Design review of the part built by this model. Coordinates are the model's own, in mm. A direction names the side the tool comes from. Give positions to 0.01 mm unless a question says otherwise; leave off trailing zeros. Loops run counter-clockwise (first coordinate to the right, second up) from the corner with the lowest first, then second, coordinate; pieces in that order, holes last. Notation, with made-up numbers: (23, 20.5) - (80, 20.5) arc R35 ccw to (80, 52.5) - close; hole circle Ø5 at (60.5, -40). An arc over 180 degrees is marked (long way). Write each question's results on one line, items separated by ' | '.
```python
from build123d import *

# Parameters (mm, degrees)
SKETCH1_R           = 24
SKETCH1_R_2         = 1.2
BOSS_EXTRUDE1_DEPTH = 1.2
SKETCH2_R           = 24
SKETCH2_R_2         = 15
BOSS_EXTRUDE2_DEPTH = 15
SKETCH3_R           = 24
SKETCH3_R_2         = 21.5
BOSS_EXTRUDE3_DEPTH = 2.4
SKETCH5_R           = 12
CUT_EXTRUDE2_DEPTH  = 20
SKETCH6_R           = 20
SKETCH6_R_2         = 19
CUT_EXTRUDE3_DEPTH  = 1.6


with BuildPart() as part:
    # Sketch1 → Boss-Extrude1 (new body)
    with BuildSketch(Plane(origin=(0, 0, 0), x_dir=(1, 0, 0), z_dir=(0, 1, 0))):
        with Locations(Location((0, 0, 0), (0, 0, 270))):
            Circle(SKETCH1_R)
        with Locations(Location((4.242640687, 4.242640687, 0), (0, 0, 270))):
            Circle(SKETCH1_R_2, mode=Mode.SUBTRACT)
        with Locations(Location((-4.242640687, 4.242640687, 0), (0, 0, 270))):
            Circle(SKETCH1_R_2, mode=Mode.SUBTRACT)
        with Locations(Location((4.242640687, -4.242640687, 0), (0, 0, 270))):
            Circle(SKETCH1_R_2, mode=Mode.SUBTRACT)
        with Locations(Location((-4.242640687, -4.242640687, 0), (0, 0, 270))):
            Circle(SKETCH1_R_2, mode=Mode.SUBTRACT)
    extrude(amount=BOSS_EXTRUDE1_DEPTH)

    # Sketch2 → Boss-Extrude2 (add)
    with BuildSketch(Plane(origin=(0, 1.2, 0), x_dir=(1, 0, 0), z_dir=(0, 1, 0))):
        with Locations(Location((0, 0, 0), (0, 0, 270))):
            Circle(SKETCH2_R)
        with Locations(Location((0, 0, 0), (0, 0, 270))):
            Circle(SKETCH2_R_2, mode=Mode.SUBTRACT)
    extrude(amount=BOSS_EXTRUDE2_DEPTH)

    # Sketch3 → Boss-Extrude3 (add)
    with BuildSketch(Plane(origin=(0, 16.2, 0), x_dir=(1, 0, 0), z_dir=(0, 1, 0))):
        with Locations(Location((0, 0, 0), (0, 0, 270))):
            Circle(SKETCH3_R)
        with Locations(Location((0, 0, 0), (0, 0, 270))):
            Circle(SKETCH3_R_2, mode=Mode.SUBTRACT)
    extrude(amount=BOSS_EXTRUDE3_DEPTH)

    # Sketch5 → Cut-Extrude2 (cut)
    with BuildSketch(Plane.XY.offset(24)):
        with Locations((0, 14)):
            Circle(SKETCH5_R)
    extrude(amount=-CUT_EXTRUDE2_DEPTH, mode=Mode.SUBTRACT)

    # Sketch6 → Cut-Extrude3 (cut)
    with BuildSketch(Plane.XZ):
        with Locations(Location((0, 0, 0), (0, 0, 270))):
            Circle(SKETCH6_R)
        with Locations(Location((0, 0, 0), (0, 0, 270))):
            Circle(SKETCH6_R_2, mode=Mode.SUBTRACT)
    extrude(amount=-CUT_EXTRUDE3_DEPTH, mode=Mode.SUBTRACT)


solid = part.part
```
Item 1: We need section B-B on z = 0. Give the boundary of the cut face in (x, y).
Output values:
outline: (-24, 0) - (-20, 0) - (-20, 1.6) - (-19, 1.6) - (-19, 0) - (19, 0) - (19, 1.6) - (20, 1.6) - (20, 0) - (24, 0) - (24, 18.6) - (21.5, 18.6) - (21.5, 16.2) - (15, 16.2) - (15, 1.2) - (-15, 1.2) - (-15, 16.2) - (-21.5, 16.2) - (-21.5, 18.6) - (-24, 18.6) - close
Item 2: We need section D-D on x = 17. Give the boundary of the cut face in (y, z).
Output values:
outline: (0, -16.94) - (18.6, -16.94) - (18.6, -13.16) - (16.2, -13.16) - (16.2, 13.16) - (18.6, 13.16) - (18.6, 16.94) - (0, 16.94) - (0, 10.54) - (1.6, 10.54) - (1.6, 8.49) - (0, 8.49) - (0, -8.49) - (1.6, -8.49) - (1.6, -10.54) - (0, -10.54) - close
Item 3: Clearance check with flat-ended pins moving along their axes: P1, Ø6, axis at y = 11, z = -5, coming from the +X side; P2, Ø4, axis at x = -14.5, z = -12.5, coming from the +Y side; P3, Ø5, axis at y = 7, z = 4, coming from the +X side. State where each tip first meets the part, or that it passes through.
Output values:
P1: stops at x = 23.92 | P2: stops at y = 16.2 | P3: stops at x = 23.95
Item 4: Tool access review of faces 4 (the face through (-7, 1.6, -18)), 5 (the face through (0, 2, 17)), 6 (the face through (3, 16.2, -15)), 7 (the face through (5.254, 0.592, -3.598)): name each direction out of +Z, -Z, +X, -X, +Y, -Y from which nothing blocks a thin tool from reaching the whole face with its end or side.
Output values:
face 4: -Y | face 5: +Z | face 6: +Y | face 7: +Y, -Y
Item 5: We need section C-C on y = 10.25. Give the boundary of the cut face in (x, z), then the cut area to 3 significant figures.
Output values:
outline: (-11.4, 9.75) - (-11.4, 21.12) arc R24 ccw (long way) to (11.4, 21.12) - (11.4, 9.75) arc R15 cw (long way) to start | area: 882 mm²
Item 6: Wall thickness on probe 1 along X at (y, z) = (0.9, 0); probe 2 along X at (y, z) = (11.5, 0); probe 3 along Y at (x, z) = (-10.5, -15): over which ranges is each line inside the solid? List them lowest first.
Output values:
probe 1: x = -24 to -20, -19 to 19, 20 to 24 | probe 2: x = -24 to -15, 15 to 24 | probe 3: y = 0 to 16.2
Item 7: We need section A-A on x = 0. Give the boundary of the cut face in (y, z), then the cut area to 3 significant figures.
Output values:
outline: (0, -24) - (18.6, -24) - (18.6, -21.5) - (16.2, -21.5) - (16.2, -15) - (1.2, -15) - (1.2, 15) - (2, 15) - (2, 24) - (0, 24) - (0, 20) - (1.6, 20) - (1.6, 19) - (0, 19) - (0, -19) - (1.6, -19) - (1.6, -20) - (0, -20) - close | area: 203 mm²
Item 8: Draft analysis for pull direction Z (two halves, no side actions). For faces 1 (the face through (1.055, 9.17, -23.977)), 2 (the face through (20, 0, -5)), 3 (the face through (0.782, 17.383, -21.486)), state which applies: +Z half, -Z half, draft (parallel to the pull), parting line (faces both ways), or undercut.
Output values:
face 1: parting line | face 2: draft | face 3: undercut
